Autodesk Inventor part; units mm, degrees
ref_plane "Work Plane1" through (29, 0, 0) normal (0, -1, 0) x (1, 0, 0)
ref_plane "YZ Plane" through (0, 0, 0) normal (1, 0, 0) x (0, 1, 0)
ref_plane "XZ Plane" through (0, 0, 0) normal (0, 1, 0) x (-1, 0, 0)
sketch "Sketch1" plane through (0, 0, 0) normal (0, 0, 1) x (1, 0, 0)
  line L0 (0.2, 0) -> (16, 0)
  line L1 (16, 0) -> (16, 2.5)
  line L2 (16, 2.5) -> (2.4, 2.5)
  line L3 (2.4, 2.5) -> (1.9091, 2.5)
  line L4 (1.9091, 2.5) -> (0, 2.5)
  line L5 (0, 2.5) -> (0, 4.25)
  line L6 (0, 4.25) -> (-3.5, 4.25)
  line L7 (-3.5, 4.25) -> (-3.5, 1.7321)
  line L8 (-3.5, 1.7321) -> (-0.8, 1.7321)
  line L9 (-0.8, 1.7321) -> (0.2, 0)
  line L10 (-7.4, 0) -> (19.9, 0)
  line L11 (0, -0.85) -> (0, 5.1)
  line L12 (2.4, 2.5) -> (0, 2.5) construction
  dimension "d1" = 13.6
  dimension "d2" = 0.4909
  dimension "d3" = 3.5
  dimension "d4" = 2.7
  dimension "d5" = 60
  dimension "d6" = 5
  dimension "d7" = 5
  dimension "d8" = 3.4641
  dimension "d9" = 8.5
  dimension "d26" = 16
revolve "Body" add sketch "Sketch1" angle 360 about axis through (0.2, 0, 0) along (1, 0, 0) contours L9 L11 L4 L3 L2 L1 L0 | L9 L8 L7 L6 L5 L11
sketch "Sketch2" plane through (-3.5, 0, 0) normal (-1, 0, 0) x (0, 0, 1)
  circle A0 centre (0, 0) radius 1.7321
  line L0 (0, -5.95) -> (0, 5.95)
  line L1 (-5.95, 0) -> (5.95, 0)
  line L2 (1.7321, 0) -> (0.866, -1.5)
  line L3 (0.866, -1.5) -> (-0.866, -1.5)
  line L4 (-0.866, -1.5) -> (-1.7321, 0)
  line L5 (-1.7321, 0) -> (-0.866, 1.5)
  line L6 (-0.866, 1.5) -> (0.866, 1.5)
  line L7 (0.866, 1.5) -> (1.7321, 0)
extrude "Slot" add sketch "Sketch2" against normal up to next contours L7 A0 | A0 L2 | L6 L0 A0 | A0 L0 L3 | L0 L6 A0 | A0 L3 L0 | L4 A0 | A0 L5
fillet "Fillet1" radius 0.5 1 edges at (-3.5, -4.25, 0)
thread "Thread"
chamfer "Chamfer1" distance 0.4908 distance2 0.4908 1 edges at (16, -2.5, 0) measured on face at (16, -1.1374, -1.1324)
ref_plane "Work Plane1" through (29, 0, 0) normal (0, -1, 0) x (1, 0, 0)
fillet "Fillet2" radius 0.1 1 edges at (0, -2.5, 0)
equation "\"d1\" = GEL"
equation "\"d3\" = KOH"
equation "\"d4\" = INTI"
equation "\"d6\" = GD"
equation "\"d7\" = BDM"
equation "\"d8\" = 1.1547 * SW"
equation "\"d9\" = KOD"
equation "\"d26\" = NLG"
equation "\"d30\" = R"
equation "\"d17\" = RR"
equation "\"d13\" = GEL"
equation "\"d15\" = -0.5 * SPD + 0.5 * GD"
equation "\"d16\" = GUL"
equation "\"GD\" = NND"
equation "\"NLG\" = 16"
equation "\"GEL\" = 13.6"
equation "\"KOD\" = 8.5"
equation "\"KOH\" = 3.5"
equation "\"INTI\" = 2.7"
equation "\"GAL\" = 0.61345 * PTC"
equation "\"GUL\" = 0.61345 * PTC"
equation "\"BDM\" = NND"
equation "\"SW\" = 3"
equation "\"RR\" = 0.5"
equation "\"SPD\" = NND - 1.2269 * PTC"
equation "\"R\" = 0.1"
equation "\"TOA\" = 30deg"
equation "\"GD1\" = THREADDIA - 1.2269 * PTC"
equation "\"THREADDIA\" = 5"
equation "\"FAWI\" = 45deg"
equation "\"ANG\" = 120deg"
equation "\"PTC\" = 0.8"
equation "\"NND\" = 5"
equation "\"E0\" = 1.155 * SW"
properties part number "DIN 7984 - M5 x 16" material "Steel, Mild"
Model file for the job. Use its own axes, mm. A direction names the side the tool comes from. Give positions to 0.01 mm unless a question says otherwise; leave off trailing zeros. Loops run counter-clockwise (first coordinate to the right, second up) from the corner with the lowest first, then second, coordinate; pieces in that order, holes last. Notation, with made-up numbers: (56.5, 26) -> (99.5, 26) arc R14 ccw to (99.5, 32) -> close; hole circle Ø10 at (33, 76). An arc over 180 degrees is marked (long way). Write each question's results on one line, items separated by ' | '.
(1) Flat gauge pins, fed straight in: pin 1 Ø3 at (x, y) = (13.5, 1.5) entering from -Z; pin 2 Ø3 at (x, y) = (12, -3) entering from +Z; pin 3 Ø0.5 at (x, z) = (-2, -0.5) entering from +Y. Where does each tip first touch, or does it go through?
Geometry results:
pin 1: stops at z = -2.5 | pin 2: stops at z = 2 | pin 3: stops at y = 4.24
(2) Probe line 1 along X through (y, z) = (-2.5, -1.25); line 2 along Z through (x, y) = (5, -2); line 3 along Z through (x, y) = (1.25, 1.5). List the from-to ranges inside material, lowest first.
Geometry results:
line 1: x = -3.5 to 0 | line 2: z = -1.5 to 1.5 | line 3: z = -2 to 2
(3) Pull direction Z, two halves, no side cores. Call faces 1 (the cylindrical face through (7.7, -0.54, 2.44)), 2 (the flat face through (-2.103, -0.74, 1.305)), 3 (the conical face through (0.137, 0.05, 0.096)), 4 (the flat face through (16, 0, 0)): released by +Z, released by -Z, zero draft, split by the parting line, or undercut.
Geometry results:
face 1: split by the parting line | face 2: undercut | face 3: undercut | face 4: zero draft
(4) Tool access for faces 5 (the flat face through (-2.103, -0.761, -1.293)), 6 (the flat face through (-3.5, -2, 0)), 7 (the flat face through (0, 2, 2)): list every direction of +Z, -Z, +X, -X, +Y, -Y with a clear straight run to the whole face (end or side of a thin tool).
Geometry results:
face 5: -X | face 6: +Z, -Z, -X, +Y, -Y | face 7: +X
(5) Cut at A-A on x = 12.25. List the corners of the cut face in (y, z), and give its area (3 significant figures).
Geometry results:
outline: circle Ø5 at (0, 0) | area: 19.6 mm²
